Check sheet for the modelled part. Datum: model origin and axes. Units: mm. A direction names the side the tool comes from. Round coordinates to 2 decimals unless told otherwise and drop trailing zeros. Write each loop counter-clockwise with the first axis right and the second up, starting at its lowest first coordinate (ties: lowest second). Pieces come first, ordered by that corner, then holes. Notation, with made-up numbers: (75.5, 57) -> (122.5, 57) arc R23 cw to (122.5, 73) -> close; hole circle Ø11 at (7, 13.25). An arc over 180 degrees is marked (long way). One line per item, written item: value.
Autodesk Inventor part; units mm, degrees
ref_plane "YZ Plane" through (0, 0, 0) normal (1, 0, 0) x (0, 1, 0)
ref_plane "XZ Plane" through (0, 0, 0) normal (0, 1, 0) x (-1, 0, 0)
ref_plane "XY Plane" through (0, 0, 0) normal (0, 0, 1) x (1, 0, 0)
sketch "Sketch1" plane through (0, 0, 0) normal (0, 1, 0) x (-1, 0, 0)
  line L0 (-70.485, -70.485) -> (5.715, -70.485)
  line L1 (5.715, -70.485) -> (5.715, 5.715)
  line L2 (5.715, 5.715) -> (-70.485, 5.715)
  line L3 (-70.485, 5.715) -> (-70.485, -70.485)
  line L4 (-70.485, -70.485) -> (5.715, 5.715) construction
  line L5 (5.715, -70.485) -> (-70.485, 5.715) construction
  line L6 (5.715, 5.715) -> (0.635, 5.715) construction
  line L7 (0.635, 5.715) -> (0.635, 0.635) construction
  line L8 (0.635, 0.635) -> (5.715, 0.635) construction
  line L9 (5.715, 0.635) -> (5.715, 5.715) construction
  line L10 (-3.175, -3.175) -> (-61.595, -3.175)
  line L11 (-61.595, -3.175) -> (-61.595, -61.595)
  line L12 (-61.595, -61.595) -> (-3.175, -61.595)
  line L13 (-3.175, -61.595) -> (-3.175, -3.175)
  line L14 (-3.175, -3.175) -> (-61.595, -61.595) construction
  line L15 (-61.595, -3.175) -> (-3.175, -61.595) construction
  circle A0 centre (0.635, 0.635) radius 1.7399
  circle A1 centre (0.635, -65.405) radius 1.7399
  circle A2 centre (-65.405, 0.635) radius 1.7399
  circle A3 centre (-65.405, -65.405) radius 1.7399
  point P0 (0, 0)
  point P1 (-32.385, -32.385)
  dimension "d2" = 76.2
  dimension "d3" = 76.2
  dimension "d4" = 5.08
  dimension "d5" = 5.08
  dimension "d7" = 58.42
  dimension "d8" = 58.42
  dimension "d9" = 3.4798
  dimension "d12" = 66.04
  dimension "d15" = 66.04
extrude "Extrusion1" add sketch "Sketch1" along normal blind 22.86
sketch "Sketch2" plane through (0, 22.86, 0) normal (0, 1, 0) x (1, 0, 0)
  line L0 (-5.715, -5.715) -> (70.485, -5.715)
  line L1 (70.485, -5.715) -> (70.485, 70.485)
  line L2 (-5.715, -5.715) -> (70.485, -5.715)
  line L3 (70.485, -5.715) -> (70.485, 70.485)
  line L4 (70.485, 70.485) -> (-5.715, 70.485)
  line L5 (-5.715, 70.485) -> (-5.715, -5.715)
  point P0 (0, 0)
extrude "Extrusion2" add sketch "Sketch2" along normal blind 2.54
sketch "Sketch3" plane through (-5.715, 0, -70.485) normal (-1, 0, 0) x (0, 0, 1)
  line L0 (38.1, 0) -> (38.1, 25.4) construction
  line L1 (76.2, 25.4) -> (0, 25.4) construction
  line L2 (38.1, 0) -> (40.005, 0) construction
  line L3 (40.005, 0) -> (36.195, 0)
  line L4 (36.195, 0) -> (36.195, 1.27)
  line L5 (40.005, 1.27) -> (40.005, 0)
  arc A0 (40.005, 1.27) -> (36.195, 1.27) centre (38.1, 1.27) ccw
  point P0 (70.485, 0)
  point P1 (38.1, 3.175)
  dimension "d24" = 1.27
  dimension "d25" = 3.81
  dimension "d26" = 1.905
extrude "Extrusion3" cut sketch "Sketch3" against normal up to surface (8.89 mm away)
sketch "Sketch4" plane through (0, 0, 0) normal (0, -1, 0) x (1, 0, 0)
  line L0 (61.595, -3.175) -> (3.175, -3.175) construction
  line L1 (-5.715, 5.715) -> (70.485, 5.715) construction
  line L2 (3.175, -3.175) -> (61.595, -3.175)
  line L3 (61.595, -3.175) -> (61.595, 1.27)
  line L4 (61.595, 1.27) -> (3.175, 1.27)
  line L5 (3.175, 1.27) -> (3.175, -3.175)
  line L6 (70.485, -70.485) -> (-5.715, -70.485) construction
  circle A0 centre (32.385, -32.385) radius 4.575 construction
  line L7 (-1.27, -61.595) -> (3.175, -61.595)
  line L8 (3.175, -61.595) -> (3.175, -3.175)
  line L9 (3.175, -3.175) -> (-1.27, -3.175)
  line L10 (-1.27, -3.175) -> (-1.27, -61.595)
  line L11 (61.595, -66.04) -> (61.595, -61.595)
  line L12 (61.595, -61.595) -> (3.175, -61.595)
  line L13 (3.175, -61.595) -> (3.175, -66.04)
  line L14 (3.175, -66.04) -> (61.595, -66.04)
  line L15 (66.04, -3.175) -> (61.595, -3.175)
  line L16 (61.595, -3.175) -> (61.595, -61.595)
  line L17 (61.595, -61.595) -> (66.04, -61.595)
  line L18 (66.04, -61.595) -> (66.04, -3.175)
  point P0 (0, 0)
  dimension "d31" = 360
extrude "Extrusion4" cut sketch "Sketch4" against normal blind 22.86 contours L5 L4 L3 L2 | L8 L7 L10 L9 | L15 L18 L17 L16 | L12 L11 L14 L13
properties part number "keypad cover"
Item 1: Sectioned sample at D-D on y = 12. Enter the section's corners in (x, z) (3 decimals).
Answer:
outline: (-5.715, -70.485) -> (70.485, -70.485) -> (70.485, 5.715) -> (-5.715, 5.715) -> close; hole circle Ø3.48 at (-0.635, -65.405); hole circle Ø3.48 at (-0.635, 0.635); hole (-1.27, -61.595) -> (3.175, -61.595) -> (3.175, -66.04) -> (61.595, -66.04) -> (61.595, -61.595) -> (66.04, -61.595) -> (66.04, -3.175) -> (61.595, -3.175) -> (61.595, 1.27) -> (3.175, 1.27) -> (3.175, -3.175) -> (-1.27, -3.175) -> close; hole circle Ø3.48 at (65.405, -65.405); hole circle Ø3.48 at (65.405, 0.635)
Item 2: Mould release check, pull along X, two halves, no side actions. Record for faces 3 (the flat face through (-5.715, 13, -33)), 4 (the flat face through (32, 13, 5.715)), 5 (the flat face through (70.485, 13, -32)), 6 (the cylindrical face through (67.143, 11.27, -65.482)): pulls with the +X half, pulls with the -X half, needs draft (parallel to the pull), parting line crosses it, or undercut.
Answer:
face 3: pulls with the -X half
face 4: needs draft
face 5: pulls with the +X half
face 6: undercut
Item 3: Thickness scan on line 1 (X direction, y = 10.75, z = -24) (3 decimals); line 2 (Z direction, x = 13, y = 10.25) (3 decimals); line 3 (Z direction, x = 66, y = 7.75) (3 decimals). Record the ranges inside material, lowest first.
Answer:
line 1: x = -5.715 to -1.27, 66.04 to 70.485
line 2: z = -70.485 to -66.04, 1.27 to 5.715
line 3: z = -70.485 to -67.04, -63.77 to -61.595, -3.175 to -1, 2.27 to 5.715
Item 4: Depth check by flat-ended pin: P1, Ø4, axis at x = -1, z = 1, coming from the -Y side; P2, Ø5, axis at x = 47, z = -54.5, coming from the -Y side. Enter the tip coordinate at first touch or a pass-through.
Answer:
P1: stops at y = 0
P2: stops at y = 22.86
Item 5: Sectioned sample at A-A on x = 8.5. Enter the section's corners in (y, z) (3 decimals), and give its area (3 significant figures).
Answer:
outline: (0, -70.485) -> (25.4, -70.485) -> (25.4, 5.715) -> (0, 5.715) -> (0, 1.27) -> (22.86, 1.27) -> (22.86, -66.04) -> (0, -66.04) -> close
area: 397 mm^2
Item 6: Tool access check on faces 1 (the flat face through (-1, 22.86, -65)), 2 (the flat face through (30, 0, 2)). Record the directions out of +Z, -Z, +X, -X, +Y, -Y that give a thin tool (end or side, any length) a straight path to the whole face; none if there is none.
Answer:
face 1: -Y
face 2: +Z, -Z, +X, -X, -Y
Item 7: Sectioned sample at B-B on y = 2.25. Enter the section's corners in (x, z) (3 decimals).
Answer:
outline: (-5.715, -70.485) -> (70.485, -70.485) -> (70.485, 5.715) -> (-5.715, 5.715) -> (-5.715, -30.751) -> (-1.27, -30.751) -> (-1.27, -3.175) -> (3.175, -3.175) -> (3.175, 1.27) -> (61.595, 1.27) -> (61.595, -3.175) -> (66.04, -3.175) -> (66.04, -61.595) -> (61.595, -61.595) -> (61.595, -66.04) -> (3.175, -66.04) -> (3.175, -61.595) -> (-1.27, -61.595) -> (-1.27, -34.019) -> (-5.715, -34.019) -> close; hole circle Ø3.48 at (-0.635, -65.405); hole circle Ø3.48 at (-0.635, 0.635); hole circle Ø3.48 at (65.405, -65.405); hole circle Ø3.48 at (65.405, 0.635)
Item 8: Sectioned sample at C-C on z = -6.5. Enter the section's corners in (x, y) (3 decimals), and give its area (3 significant figures).
Answer:
outline: (-5.715, 0) -> (-1.27, 0) -> (-1.27, 22.86) -> (66.04, 22.86) -> (66.04, 0) -> (70.485, 0) -> (70.485, 25.4) -> (-5.715, 25.4) -> close
area: 397 mm^2
